from build123d import *

# Parameters (mm, degrees)
SKETCH2_W          = 3.175
SKETCH2_H          = 1.5875
CUT_EXTRUDE1_DEPTH = 130.660858204


with BuildPart() as part:
    # Sketch1 → Revolve1 (revolve)
    with BuildSketch(Plane.XY):
        Polygon((6.35, 64.16675), (5.842, 64.67475), (0, 64.67475), (0, -64.67475), (5.842, -64.67475), (6.35, -64.16675), (6.35, -61.49975), (5.08, -61.49975), (5.08, -60.22975), (6.35, -60.22975), (6.35, -48.79975), (5.08, -48.79975), (5.08, -47.52975), (6.35, -47.52975), (6.35, 8.15975), (5.08, 8.15975), (5.08, 9.42975), (6.35, 9.42975), (6.35, 34.82975), (5.08, 34.82975), (5.08, 36.09975), (6.35, 36.09975), (6.35, 60.22975), (5.08, 60.22975), (5.08, 61.49975), (6.35, 61.49975), align=None)
    revolve(axis=Axis((0, -64.67475, 0), (0, 1, 0)))

    # Sketch2 → Cut-Extrude1 (cut, through all)
    with BuildSketch(Plane(origin=(0, 64.67475, 0), x_dir=(1, 0, 0), z_dir=(0, 1, 0))):
        with Locations((0, 5.55625)):
            Rectangle(SKETCH2_W, SKETCH2_H)
    extrude(amount=-CUT_EXTRUDE1_DEPTH, mode=Mode.SUBTRACT)


solid = part.part
Design review of the part built by this model. Coordinates are the model's own, in mm. A direction names the side the tool comes from. Round coordinates to 2 decimals unless told otherwise and drop trailing zeros. Order: outer loops, then holes, each group sorted by start corner. A loop starts at its lowest first (then second) coordinate and runs counter-clockwise, first axis right, second up.
1) Consider section A-A (x = 0). State the section outline as (y, z) points.
The answers:
outline: (-64.67, -4.76) - (64.67, -4.76) - (64.67, 5.84) - (64.17, 6.35) - (61.5, 6.35) - (61.5, 5.08) - (60.23, 5.08) - (60.23, 6.35) - (36.1, 6.35) - (36.1, 5.08) - (34.83, 5.08) - (34.83, 6.35) - (9.43, 6.35) - (9.43, 5.08) - (8.16, 5.08) - (8.16, 6.35) - (-47.53, 6.35) - (-47.53, 5.08) - (-48.8, 5.08) - (-48.8, 6.35) - (-60.23, 6.35) - (-60.23, 5.08) - (-61.5, 5.08) - (-61.5, 6.35) - (-64.17, 6.35) - (-64.67, 5.84) - close
2) Machinability: for faces 1 (the conical face through (-0.24, 64.54, 5.97)), 2 (the flat face through (0, 1, -4.762)), 3 (the flat face through (-0.9, -60.23, 5.2)), which of the approach directions +Z, -Z, +X, -X, +Y, -Y give a long, thin tool a straight path to every point of the face, cutting with its end or side? Answer none if there is none.
The answers:
face 1: +Y
face 2: -Z, +Y, -Y
face 3: none
3) Draft analysis for pull direction Y (two halves, no side actions). For faces 4 (the flat face through (0, -64.675, 0)), 5 (the flat face through (0.9, -61.5, 5.2)), 6 (the cylindrical face through (-0.257, 22.308, 6.345)), state which applies: released by +Y, released by -Y, zero draft, split by the parting line, or undercut.
The answers:
face 4: released by -Y
face 5: undercut
face 6: zero draft
4) Clearance check with flat-ended pins moving along their axes: pin 1 Ø2 at (y, z) = (-5, 5) entering from -X; pin 2 Ø1.5 at (x, y) = (3.5, 15.5) entering from +Z; pin 3 Ø6 at (x, y) = (4, 19.5) entering from +Z. State where each tip first meets the part, or that it passes through.
The answers:
pin 1: stops at x = -4.93
pin 2: stops at z = 5.72
pin 3: stops at z = 6.27
5) For L1, parallel to Y at x = 3.5, z = -3.75; L2, parallel to Z at x = 0, y = 36.5; L3, parallel to Z at x = 2.5, y = 27, list the stretches that pass through material, from the lowest coordinate up.
The answers:
L1: y = -64.67 to -61.5, -60.23 to -48.8, -47.53 to 8.16, 9.43 to 34.83, 36.1 to 60.23, 61.5 to 64.67
L2: z = -4.76 to 6.35
L3: z = -5.84 to 5.84
6) Consider section B-B (y = 2.5). State the section outline as (x, z) points.
The answers:
outline: (-1.59, -6.15) - (-1.59, -4.76) - (1.59, -4.76) - (1.59, -6.15) arc R6.35 ccw (long way) to start
